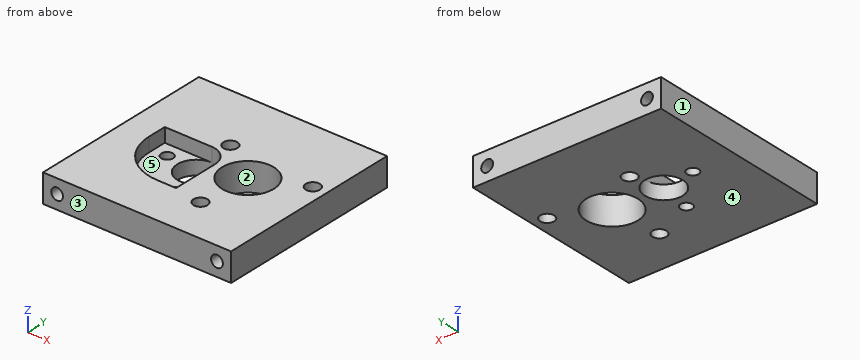
from build123d import *

# Parameters (mm, degrees)
SKETCH1_W          = 40
SKETCH1_H          = 40
EXTRUDE1_DEPTH     = 6
SKETCH8_R          = 5.5
CUT_EXTRUDE6_DEPTH = 6
SKETCH5_R          = 1.5
CUT_EXTRUDE4_DEPTH = 6
CIRPATTERN1_COUNT  = 3
EXTRUDE15_DEPTH    = 3
SKETCH35_R         = 1.25
EXTRUDE17_DEPTH    = 3
SKETCH34_R         = 4
EXTRUDE16_DEPTH    = 3
SKETCH27_R         = 1.25
EXTRUDE6_DEPTH     = 10
EXTRUDE18_START    = -10
SKETCH36_R         = 1.25
EXTRUDE18_DEPTH    = 10


# Read off the part's stored shape, not the designer's step: M3 Tapped Hole1
with BuildPart() as part:
    # Sketch1 → Extrude1 (new body)
    with BuildSketch(Plane.XY):
        with Locations((4, 0)):
            Rectangle(SKETCH1_W, SKETCH1_H)
    extrude(amount=-EXTRUDE1_DEPTH)

    # Sketch8 → Cut-Extrude6 (cut)
    with BuildSketch(Plane(origin=(0, 0, -6), x_dir=(-1, 0, 0), z_dir=(0, 0, -1))):
        with Locations((-11, 0)):
            Circle(SKETCH8_R)
    extrude(amount=-CUT_EXTRUDE6_DEPTH, mode=Mode.SUBTRACT)

    # Sketch5 → Cut-Extrude4 (cut)
    with BuildSketch(Plane(origin=(0, 0, -6), x_dir=(-1, 0, 0), z_dir=(0, 0, -1))):
        with Locations((-10, -10.95445115)):
            Circle(SKETCH5_R)
    cut_extrude4 = extrude(amount=-CUT_EXTRUDE4_DEPTH, mode=Mode.SUBTRACT)

    # CirPattern1: Cut-Extrude4 ×3 about axis
    cirpattern1_axis = Axis((11, 0, 0), (0, 0, 1))
    for i in range(1, CIRPATTERN1_COUNT):
        add(cut_extrude4.rotate(cirpattern1_axis, i * 360 / CIRPATTERN1_COUNT), mode=Mode.SUBTRACT)

    # Sketch29 → Extrude15 (cut)
    with BuildSketch(Plane.XY):
        with BuildLine():
            Line((4, 0), (4, -10))
            Line((4, -10), (0, -10))
            ThreePointArc((0, -10), (-7.071067812, -7.071067812), (-10, 0))
            Line((-10, 0), (-10, 4))
            Line((-10, 4), (0, 4))
            ThreePointArc((0, 4), (2.828427125, 2.828427125), (4, 0))
        make_face()
    extrude(amount=-EXTRUDE15_DEPTH, mode=Mode.SUBTRACT)

    # Sketch35 → Extrude17 (cut)
    with BuildSketch(Plane.XY.offset(-3)):
        with Locations((1, -7)):
            Circle(SKETCH35_R)
        with Locations((-7, 1)):
            Circle(SKETCH35_R)
    extrude(amount=-EXTRUDE17_DEPTH, mode=Mode.SUBTRACT)

    # Sketch34 → Extrude16 (cut)
    with BuildSketch(Plane.XY.offset(-3)):
        Circle(SKETCH34_R)
    extrude(amount=-EXTRUDE16_DEPTH, mode=Mode.SUBTRACT)

    # Sketch27 → Extrude6 (cut)
    with BuildSketch(Plane(origin=(0, 20, 0), x_dir=(1, 0, 0), z_dir=(0, 1, 0))):
        with Locations(Location((-13, 3, 0), (0, 0, 180))):
            Circle(SKETCH27_R)
        with Locations(Location((21, 3, 0), (0, 0, 180))):
            Circle(SKETCH27_R)
    extrude(amount=-EXTRUDE6_DEPTH, mode=Mode.SUBTRACT)

    # Sketch36 → Extrude18 (cut)
    with BuildSketch(Plane.XZ.offset(20).offset(EXTRUDE18_START)):
        with Locations(Location((-13, -3, 0), (0, 0, 180))):
            Circle(SKETCH36_R)
        with Locations(Location((21, -3, 0), (0, 0, 180))):
            Circle(SKETCH36_R)
    extrude(amount=EXTRUDE18_DEPTH, mode=Mode.SUBTRACT)

    # M3 Tapped Hole1 outline → M3 Tapped Hole1 (revolve, cut)
    with BuildSketch(Plane(origin=(21, 0, -3), x_dir=(1, 0, 0), z_dir=(0, 0, 1))):
        Polygon((1.25, -10), (0, -9.248924226), (0, -10), align=None)
        Polygon((0, 10), (0, 9.248924226), (1.25, 10), align=None)
    revolve(axis=Axis((21, 0, -3), (0, 1, 0)), mode=Mode.SUBTRACT)

    # M3 Tapped Hole1 2 outline → M3 Tapped Hole1 2 (revolve, cut)
    with BuildSketch(Plane(origin=(-13, 0, -3), x_dir=(1, 0, 0), z_dir=(0, 0, 1))):
        Polygon((1.25, -10), (0, -9.248924226), (0, -10), align=None)
        Polygon((0, 10), (0, 9.248924226), (1.25, 10), align=None)
    revolve(axis=Axis((-13, 0, -3), (0, 1, 0)), mode=Mode.SUBTRACT)


solid = part.part
Here's how the part is built. I have some questions about the finished solid (model axes, mm). Face numbers are marked on the shaded views. A direction names the side the tool comes from. Round coordinates to 2 decimals unless told otherwise and drop trailing zeros. Write each loop counter-clockwise with the first axis right and the second up, starting at its lowest first coordinate (ties: lowest second). Pieces come first, ordered by that corner, then holes. Notation, with made-up numbers: (6.5, -9) -> (48.5, -9) arc R12 cw to (48.5, 1) -> close; hole circle Ø2 at (-18.5, 3). An arc over 180 degrees is marked (long way). One line per item, written item: value.
1) If I drill on line 1 (X direction, y = -15.25, z = -3); line 2 (X direction, y = -12.25, z = -3); line 3 (Y direction, x = 10, z = -2.05), over which ranges is the centre line in solid material (lowest first)? Write a range as [from, to].
Filled sheet:
line 1: x = [-16, -14.25], [-11.75, 19.75], [22.25, 24]
line 2: x = [-16, -14.25], [-11.75, 9.24], [10.76, 19.75], [22.25, 24]
line 3: y = [-20, -12.45], [-9.45, -5.41], [5.41, 20]
2) For the marked faces 4 and 5, which set-ups out of +Z, -Z, +X, -X, +Y, -Y let a thin tool reach every point of the face, with its end or its side?
Filled sheet:
face 4: -Z, +X, -X, +Y, -Y
face 5: +Z
3) Suppose I cut it at D-D on y = 1. List the corners of the cut face in (x, z) for me, plus the area to 3 significant figures.
Filled sheet:
outline: (-16, -6) -> (-8.25, -6) -> (-8.25, -3) -> (-10, -3) -> (-10, 0) -> (-16, 0) -> close; (-5.75, -6) -> (-3.87, -6) -> (-3.87, -3) -> (-5.75, -3) -> close; (3.87, -6) -> (5.59, -6) -> (5.59, 0) -> (3.87, 0) -> close; (16.41, -6) -> (24, -6) -> (24, 0) -> (16.41, 0) -> close
area: 103 mm2
4) Suppose I cut it at B-B on y = -7. List the corners of the cut face in (x, z) for me.
Filled sheet:
outline: (-16, -6) -> (-0.25, -6) -> (-0.25, -3) -> (-7.14, -3) -> (-7.14, 0) -> (-16, 0) -> close; (2.25, -6) -> (24, -6) -> (24, 0) -> (4, 0) -> (4, -3) -> (2.25, -3) -> close
5) I'm going to push flat-ended pins straight in: pin 1 Ø2 at (x, z) = (21, -3) entering from +Y; pin 2 Ø1.5 at (x, z) = (-13, -3) entering from -Y. Where does each tip first touch, or does it pass through?
Filled sheet:
pin 1: stops at y = 9.85
pin 2: stops at y = -9.7
6) Suppose I cut it at C-C on z = -5.2. List the corners of the cut face in (x, y) for me.
Filled sheet:
outline: (-16, -20) -> (24, -20) -> (24, 20) -> (-16, 20) -> close; hole circle Ø2.5 at (-7, 1); hole circle Ø8 at (0, 0); hole circle Ø2.5 at (1, -7); hole circle Ø3 at (2.01, 6.34); hole circle Ø11 at (11, 0); hole circle Ø3 at (10, -10.95); hole circle Ø3 at (20.99, 4.61)
7) We'd pull the mould along Y, two halves only. Please class the marked faces 1, 2 and 3: released by +Y, released by -Y, zero draft, split by the parting line, or undercut.
Filled sheet:
face 1: zero draft
face 2: undercut
face 3: released by -Y
8) Suppose I cut it at A-A on x = 6.5. List the corners of the cut face in (y, z) for me.
Filled sheet:
outline: (-20, -6) -> (-3.16, -6) -> (-3.16, 0) -> (-20, 0) -> close; (3.16, -6) -> (20, -6) -> (20, 0) -> (3.16, 0) -> close
